from build123d import *

# Parameters (mm, degrees)
PAD_DEPTH    = 3
SKETCH001_R  = 5
PAD001_DEPTH = 5
SKETCH002_W  = 6
SKETCH002_H  = 4
POCKET_DEPTH = 5


with BuildPart() as part:
    # Sketch → Pad (new body)
    with BuildSketch(Plane.XY):
        with BuildLine():
            Line((42, -39), (42, 39))
            ThreePointArc((42, 39), (41.1213203436, 41.1213203436), (39, 42))
            Line((39, 42), (-39, 42))
            ThreePointArc((-39, 42), (-41.1213203436, 41.1213203436), (-42, 39))
            Line((-42, 39), (-42, -39))
            ThreePointArc((-42, -39), (-41.1213203436, -41.1213203436), (-39, -42))
            Line((-39, -42), (39, -42))
            ThreePointArc((39, -42), (41.1213203436, -41.1213203436), (42, -39))
        make_face()
        with BuildLine():
            Line((-15, 42), (15, 42))
            Line((15, 42), (15, 49))
            ThreePointArc((15, 49), (14.1213203436, 51.1213203436), (12, 52))
            Line((12, 52), (-12, 52))
            ThreePointArc((-12, 52), (-14.1213203436, 51.1213203436), (-15, 49))
            Line((-15, 49), (-15, 42))
        make_face()
        with BuildLine():
            Line((-15, -42), (-15, -49))
            ThreePointArc((-15, -49), (-14.1213203436, -51.1213203436), (-12, -52))
            Line((-12, -52), (12, -52))
            ThreePointArc((12, -52), (14.1213203436, -51.1213203436), (15, -49))
            Line((15, -49), (15, -42))
            Line((15, -42), (-15, -42))
        make_face()
    extrude(amount=PAD_DEPTH)

    # Sketch001 (on Face22 of Pad) → Pad001 (join)
    with BuildSketch(Plane.XY.offset(3)):
        with Locations((-30, 30)):
            Circle(SKETCH001_R)
        with Locations((-10, 30)):
            Circle(SKETCH001_R)
        with Locations((-30, 10)):
            Circle(SKETCH001_R)
        with Locations((-10, 10)):
            Circle(SKETCH001_R)
        with Locations((-30, -10)):
            Circle(SKETCH001_R)
        with Locations((-10, -10)):
            Circle(SKETCH001_R)
        with Locations((-30, -30)):
            Circle(SKETCH001_R)
        with Locations((-10, -30)):
            Circle(SKETCH001_R)
        with Locations((10, 30)):
            Circle(SKETCH001_R)
        with Locations((30, 30)):
            Circle(SKETCH001_R)
        with Locations((10, 10)):
            Circle(SKETCH001_R)
        with Locations((30, 10)):
            Circle(SKETCH001_R)
        with Locations((10, -10)):
            Circle(SKETCH001_R)
        with Locations((30, -10)):
            Circle(SKETCH001_R)
        with Locations((10, -30)):
            Circle(SKETCH001_R)
        with Locations((30, -30)):
            Circle(SKETCH001_R)
    extrude(amount=PAD001_DEPTH)

    # Sketch002 (on Face5 of Pad001) → Pocket (cut)
    with BuildSketch(Plane.XY.offset(3)):
        with Locations((-7, 47)):
            Rectangle(SKETCH002_W, SKETCH002_H)
        with Locations((7, 47)):
            Rectangle(SKETCH002_W, SKETCH002_H)
        with Locations((7, -47)):
            Rectangle(SKETCH002_W, SKETCH002_H)
        with Locations((-7, -47)):
            Rectangle(SKETCH002_W, SKETCH002_H)
    extrude(amount=-POCKET_DEPTH, mode=Mode.SUBTRACT)


solid = part.part
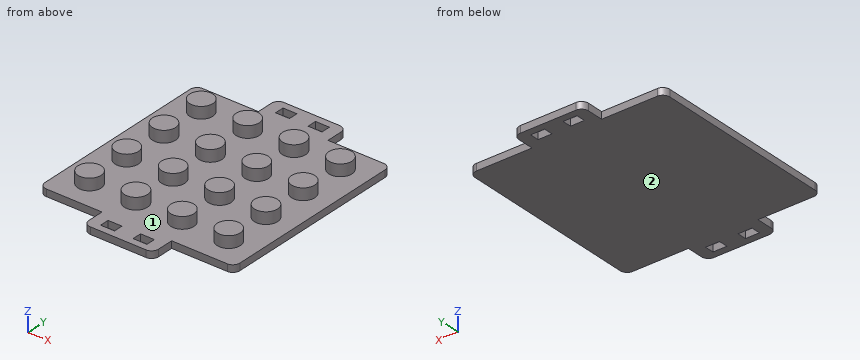
Geometry check sheet. Reference: the model listing, model coordinates, mm. Face numbers are marked on the shaded views. Give positions to 0.01 mm unless a question says otherwise; leave off trailing zeros. Loops run counter-clockwise (first coordinate to the right, second up) from the corner with the lowest first, then second, coordinate; pieces in that order, holes last. Notation, with made-up numbers: (57, -1.5) -> (76, -1.5) arc R15 ccw to (76, 13.5) -> close; hole circle Ø6 at (7, -18.5). An arc over 180 degrees is marked (long way). Answer in a Markdown table with one row per item. Add a question column.
1) Cross-section at B-B on x = 30. Record the boundary of the cut face in (y, z).
2) Gauge pin test, flat ends, axial feed: P1, Ø2.5, axis at y = 45, z = 1, coming from the +X side; P2, Ø2.5, axis at y = -45, z = 2, coming from the -X side; P3, Ø3.5, axis at x = 29.5, z = 2, coming from the +Y side. Record the tip position at first contact, or that the pin passes through.
3) Cross-section at A-A on z = 5.5. State how many separate pieces and enclosed holes the cut face has, and give its area (3 significant figures).
4) Draft check along Y on the marked faces 1 and 2. Enter one of: pulls with the +Y half, pulls with the -Y half, needs draft (parallel to the pull), parting line crosses it, or undercut.
5) Material ranges on probe 1 along Y at (x, z) = (-11, 4); probe 2 along Z at (x, y) = (-2.5, -11); probe 3 along Y at (x, z) = (19, 2.5), recorded low to high. Write a range as from..to.
6) Cross-section at D-D on x = -18. Record the boundary of the cut face in (y, z), and give its area (3 significant figures).
Outcome:
| question | item | result |
|---|---|---|
| 1 | outline | (-42, 0) -> (42, 0) -> (42, 3) -> (35, 3) -> (35, 8) -> (25, 8) -> (25, 3) -> (15, 3) -> (15, 8) -> (5, 8) -> (5, 3) -> (-5, 3) -> (-5, 8) -> (-15, 8) -> (-15, 3) -> (-25, 3) -> (-25, 8) -> (-35, 8) -> (-35, 3) -> (-42, 3) -> close |
| 2 | P1 | stops at x = 15 |
| 2 | P2 | stops at x = -15 |
| 2 | P3 | stops at y = 42 |
| 3 | separate pieces | 16 |
| 3 | enclosed holes | 0 |
| 3 | area | 1,260 mm^2 |
| 4 | face 1 | undercut |
| 4 | face 2 | needs draft |
| 5 | probe 1 | y = -34.9..-25.1, -14.9..-5.1, 5.1..14.9, 25.1..34.9 |
| 5 | probe 2 | z = 0..3 |
| 5 | probe 3 | y = -42..42 |
| 6 | outline | (-42, 0) -> (42, 0) -> (42, 3) -> (-42, 3) -> close |
| 6 | area | 252 mm^2 |
